Here's the drawing with two shaded views (mm, measured from the low corner). I have some questions. Round coordinates to 2 decimals unless told otherwise and drop trailing zeros. Order: outer loops, then holes, each group sorted by start corner. A loop starts at its lowest first (then second) coordinate and runs counter-clockwise, first axis right, second up. Notation, with made-up numbers: M 51,-28.5 L 99,-28.5 A11 ccw 99,-24.5 Z; hole C -30.75,36 d1. An arc over 180 degrees is marked long. One line per question, with ' | ' between items.
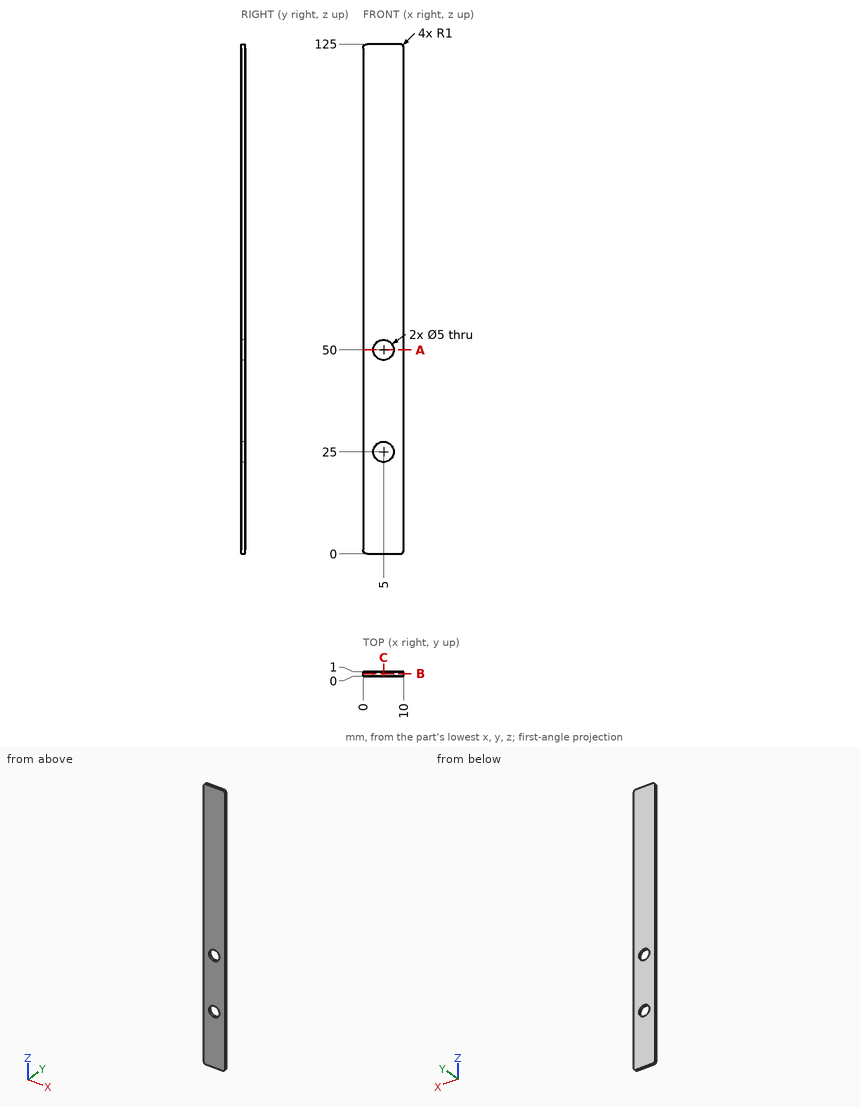
(1) Will this pin go through, and if not, where does the flat tip stop? pin 1 Ø4 at (x, z) = (5, 50) entering from +Y.
Final values:
pin 1: through
(2) If we section it at B-B on y = 0.6: Please give me the cut outline in (x, z), plus the area to 3 significant figures.
Final values:
outline: M 0,1 A1 ccw 1,0 L 9,0 A1 ccw 10,1 L 10,124 A1 ccw 9,125 L 1,125 A1 ccw 0,124 Z; hole C 5,25 d5; hole C 5,50 d5 | area: 1,210 mm^2
(3) If we section it at C-C on x = 5: Please give me the cut outline in (y, z).
Final values:
outline: M 0,0 L 1,0 L 1,22.5 L 0,22.5 Z; M 0,27.5 L 1,27.5 L 1,47.5 L 0,47.5 Z; M 0,52.5 L 1,52.5 L 1,125 L 0,125 Z
(4) If we section it at A-A on z = 50: Please give me the cut outline in (x, y), plus the area to 3 significant figures.
Final values:
outline: M 0,0 L 2.5,0 L 2.5,1 L 0,1 Z; M 7.5,0 L 10,0 L 10,1 L 7.5,1 Z | area: 5.00 mm^2
(5) Please list where these lines run through material, in increasing order: probe 1 along Z at (x, y) = (5, 0.8); probe 2 along Z at (x, y) = (4.25, 0.3). Write a range as [from, to].
Final values:
probe 1: [0, 22.5], [27.5, 47.5], [52.5, 125] | probe 2: [0, 22.62], [27.38, 47.62], [52.38, 125]
